```python
from build123d import *

# Parameters (mm, degrees)
F0_R      = 16
F1_DEPTH  = 50
F3_DEPTH  = 20
F4_W      = 60
F4_H      = 10
F5_DEPTH  = 20
F6_W      = 60
F6_H      = 10
F7_DEPTH  = 60
F8_R      = 29.99999
F9_R      = 10
F10_DEPTH = 10
F11_R     = 6
F12_DEPTH = 20.001
F14_R     = 5
F15_DEPTH = 25


# Not quite as in the source:
# - a fillet or chamfer is up to 0.001 mm smaller than in the source, because OpenCascade refuses the exact size


with BuildPart() as f1:
    # F0 (on Top) → F1 (new body)
    with BuildSketch(Plane.XY):
        with Locations((-36.3172069192, -31.1424750835)):
            Circle(F0_R)
    extrude(amount=F1_DEPTH)

    # F2 (on face) → F3 (join)
    with BuildSketch(Plane.XY.offset(50)):
        Polygon((-66.3172069192, -3.6424750835), (-66.3172069192, -31.1424750835), (-66.3172069192, -58.6424750835), (-36.3172069192, -58.6424750835), (-6.3172069192, -58.6424750835), (-6.3172069192, -31.1424750835), (-6.3172069192, -3.6424750835), (-36.3172069192, -3.6424750835), align=None)
    extrude(amount=F3_DEPTH)

    # F4 (on face) → F5 (join)
    with BuildSketch(Plane.XY.offset(70)):
        with Locations((-36.3172069192, 1.3575249165)):
            Rectangle(F4_W, F4_H)
    extrude(amount=-F5_DEPTH)

    # F6 (on face) → F7 (join)
    with BuildSketch(Plane.XY.offset(70)):
        with Locations((-36.3172069192, 1.3575249165)):
            Rectangle(F6_W, F6_H)
    extrude(amount=F7_DEPTH)

    # F8 (radius 30 in the source; OpenCascade refuses exactly that, so slightly less here)
    f8_edges = [f1.edges().sort_by_distance(p)[0] for p in [
        (-66.317207, 1.357525, 130),
        (-6.317207, 1.357525, 130),
    ]]
    fillet(f8_edges, radius=F8_R)

    # F9 (on face) → F10 (join)
    with BuildSketch(Plane.XZ.offset(3.6424750835)):
        with Locations((-36.3172069192, 100)):
            Circle(F9_R)
    extrude(amount=F10_DEPTH)

    # F11 (on face) → F12 (cut, through all)
    with BuildSketch(Plane.XZ.offset(13.6424750835)):
        with Locations((-36.3172069192, 100)):
            Circle(F11_R)
    extrude(amount=-F12_DEPTH, mode=Mode.SUBTRACT)

    # F14
    f14_edges = [f1.edges().sort_by_distance(p)[0] for p in [
        (-66.317207, -58.642475, 60),
        (-66.317207, -26.142475, 50),
        (-36.317207, -58.642475, 50),
        (-6.317207, -26.142475, 50),
        (-6.317207, -58.642475, 60),
        (-6.317207, -31.142475, 70),
    ]]
    fillet(f14_edges, radius=F14_R)

    # F6 (on face) → F15 (join)
    with BuildSketch(Plane.XY.offset(70)):
        with Locations((-36.3172069192, 1.3575249165)):
            Rectangle(F6_W, F6_H)
    extrude(amount=F15_DEPTH)


solid = f1.part
```
Read the model definition and answer for the solid it produces. Units are mm, in the model's axes. A direction names the side the tool comes from. Coordinates: 2 decimals unless noted, no trailing zeros. Write each loop counter-clockwise with the first axis right and the second up, starting at its lowest first coordinate (ties: lowest second). Pieces come first, ordered by that corner, then holes. Notation, with made-up numbers: (50.5, 45.25) -> (96.5, 45.25) arc R17 ccw to (96.5, 58.25) -> close; hole circle Ø7 at (73, 80.5). An arc over 180 degrees is marked (long way). Return JSON: item names as keys, results as strings.
1. Find the intervals of material crossed by line 1 along X through (y, z) = (-8, 100); line 2 along Y through (x, z) = (-33, 107.5); line 3 along X through (y, z) = (-3.25, 100), in increasing order. Write a range as from..to.
Found:
{"line 1": "-46.32..-42.32, -30.32..-26.32", "line 2": "-13.64..6.36", "line 3": "-66.32..-42.32, -30.32..-6.32"}
2. Determine the mould class of faces 1 (the face through (-37, 6.358, 89)), 2 (the face through (-37.1, -3.78, 105.95)), 3 (the face through (-66.317, -17, 67)), 4 (the face through (-14.872, 1.428, 120.979)) for opening direction X: pulls with the +X half, pulls with the -X half, needs draft (parallel to the pull), parting line crosses it, or undercut.
Found:
{"face 1": "needs draft", "face 2": "undercut", "face 3": "pulls with the -X half", "face 4": "pulls with the +X half"}
3. A cutting plane is placed at D-D (y = -25). Determine the outline of the cut face in (x, z).
Found:
{"outline": "(-66.32, 55) arc R5 ccw to (-61.32, 50) -> (-51.09, 50) -> (-51.09, 0) -> (-21.54, 0) -> (-21.54, 50) -> (-11.32, 50) arc R5 ccw to (-6.32, 55) -> (-6.32, 65) arc R5 ccw to (-11.32, 70) -> (-66.32, 70) -> close"}
4. Each of these flat-tipped pins is pushed along its axis until it touches: P1, Ø5, axis at x = -43.5, y = -47.5, coming from the +Z side; P2, Ø1.5, axis at x = -33, z = 26.5, coming from the -Y side; P3, Ø1, axis at x = -53, y = -8, coming from the -Z side; P4, Ø7, axis at x = -36.32, z = 100, coming from the +Y side. Where does it stop, or does it pass through?
Found:
{"P1": "z = 70", "P2": "y = -46.94", "P3": "z = 50", "P4": "through"}
5. A tool of negligible diameter and unlimited length cuts with its end or side. For faces 5 (the face through (-30, -13.642, 100)), 6 (the face through (-7.821, -30.757, 68.574)), 7 (the face through (-28.934, -45.337, 24.65)), 8 (the face through (-37.619, -8.572, 109.915)), from which of +Z, -Z, +X, -X, +Y, -Y can it reach the whole face along a straight path? Write none if from no direction.
Found:
{"face 5": "+Z, +X, -X, -Y", "face 6": "+Z, +X, -Y", "face 7": "-Z", "face 8": "-Y"}
6. A cutting plane is placed at A-A (y = -11). Determine the outline of the cut face in (x, z).
Found:
{"outline": "(-66.32, 55) arc R5 ccw to (-61.32, 50) -> (-11.32, 50) arc R5 ccw to (-6.32, 55) -> (-6.32, 65) arc R5 ccw to (-11.32, 70) -> (-66.32, 70) -> close; circle Ø20 at (-36.32, 100); hole circle Ø12 at (-36.32, 100)"}
7. A cutting plane is placed at C-C (x = -35). Determine the outline of the cut face in (y, z).
Found:
{"outline": "(-58.64, 55) arc R5 ccw to (-53.64, 50) -> (-47.09, 50) -> (-47.09, 0) -> (-15.2, 0) -> (-15.2, 50) -> (6.36, 50) -> (6.36, 95) -> (-3.64, 95) -> (-3.64, 94.15) -> (-13.64, 94.15) -> (-13.64, 90.09) -> (-3.64, 90.09) -> (-3.64, 70) -> (-58.64, 70) -> close; (-13.64, 105.85) -> (6.36, 105.85) -> (6.36, 129.97) -> (-3.64, 129.97) -> (-3.64, 109.91) -> (-13.64, 109.91) -> close"}
8. A cutting plane is placed at B-B (z = 104). Determine the outline of the cut face in (x, y), and give its area (3 significant figures).
Found:
{"outline": "(-66.05, -3.64) -> (-45.48, -3.64) -> (-45.48, -13.64) -> (-40.79, -13.64) -> (-40.79, 6.36) -> (-66.05, 6.36) -> close; (-31.85, -13.64) -> (-27.15, -13.64) -> (-27.15, -3.64) -> (-6.59, -3.64) -> (-6.59, 6.36) -> (-31.85, 6.36) -> close", "area": "599 mm2"}
